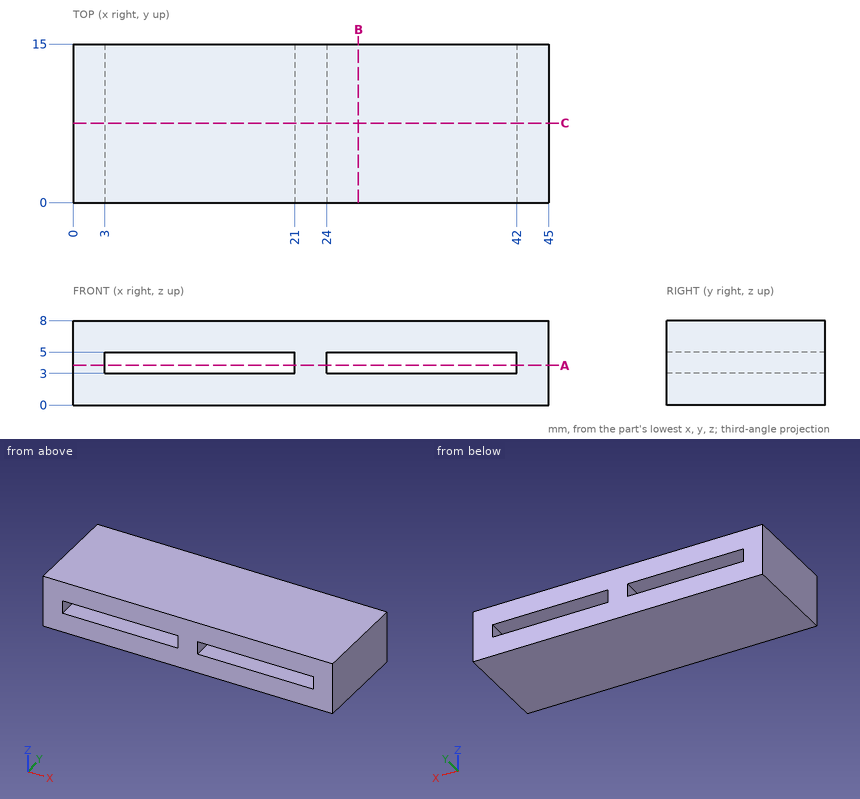
Input: dimensioned drawing with shaded views. Units: mm. Origin: part minimum x, y, z. Coordinates: 2 decimals unless noted, no trailing zeros. Loops run counter-clockwise (first coordinate to the right, second up) from the corner with the lowest first, then second, coordinate; pieces in that order, holes last. Notation, with made-up numbers: (17.5, 47.25) -> (36.5, 47.25) arc R38 cw to (36.5, 85.25) -> close; hole circle Ø6 at (-22, 30). An arc over 180 degrees is marked (long way). One line per item, written item: value. Start each with the question number.
Q1. Section query C-C, the plane y = 7.5. Return the cut outline in (x, z).
Q2. Section query A-A, the plane z = 3.75. Return the cut outline in (x, y).
Q3. Line query: line 1 along Z through (x, y) = (26, 9.25); line 2 along X through (y, z) = (12, 4.75). Output: solid intervals per line, ascending.
Q4. Section query B-B, the plane x = 27. Return the cut outline in (y, z).
Results:
1. outline: (0, 0) -> (45, 0) -> (45, 8) -> (0, 8) -> close; hole (3, 3) -> (21, 3) -> (21, 5) -> (3, 5) -> close; hole (24, 3) -> (42, 3) -> (42, 5) -> (24, 5) -> close
2. outline: (0, 0) -> (3, 0) -> (3, 15) -> (0, 15) -> close; (21, 0) -> (24, 0) -> (24, 15) -> (21, 15) -> close; (42, 0) -> (45, 0) -> (45, 15) -> (42, 15) -> close
3. line 1: 0 to 3, 5 to 8
3. line 2: 0 to 3, 21 to 24, 42 to 45
4. outline: (0, 0) -> (15, 0) -> (15, 3) -> (0, 3) -> close; (0, 5) -> (15, 5) -> (15, 8) -> (0, 8) -> close
